Part model, mm, in its own coordinate system. Face numbers are marked on the shaded views. A direction names the side the tool comes from. Coordinates: 2 decimals unless noted, no trailing zeros. Loops run counter-clockwise (first coordinate to the right, second up) from the corner with the lowest first, then second, coordinate; pieces in that order, holes last.
Autodesk Inventor part; units mm, degrees
ref_plane "YZ Plane" through (0, 0, 0) normal (1, 0, 0) x (0, 1, 0)
ref_plane "XZ Plane" through (0, 0, 0) normal (0, 1, 0) x (-1, 0, 0)
ref_plane "XY Plane" through (0, 0, 0) normal (0, 0, 1) x (1, 0, 0)
sketch "Sketch1" plane through (0, 0, 0) normal (0, 0, 1) x (1, 0, 0)
  line L0 (-34.8609, 0) -> (34.8609, 0) construction
  line L1 (0, -34.8609) -> (0, 34.8609) construction
  line L2 (0, 0) -> (13.4339, 13.4339) construction
  line L3 (0, 0) -> (18.9985, 0) construction
  line L4 (0, 24.9006) -> (16.8, 24.9006)
  line L5 (16.8, 24.9006) -> (16.8, 21.2406)
  line L6 (16.8, 21.2406) -> (19.0203, 19.0203)
  line L7 (24.9006, 0) -> (24.9006, 16.8)
  line L8 (24.9006, 16.8) -> (21.2406, 16.8)
  line L9 (21.2406, 16.8) -> (19.0203, 19.0203)
  line L10 (0, 0) -> (-13.4339, 13.4339) construction
  line L11 (0, 0) -> (-18.9985, 0) construction
  line L12 (0, 24.9006) -> (-16.8, 24.9006)
  line L13 (-16.8, 24.9006) -> (-16.8, 21.2406)
  line L14 (-16.8, 21.2406) -> (-19.0203, 19.0203)
  line L15 (-24.9006, 0) -> (-24.9006, 16.8)
  line L16 (-24.9006, 16.8) -> (-21.2406, 16.8)
  line L17 (-21.2406, 16.8) -> (-19.0203, 19.0203)
  line L18 (0, 0) -> (13.4339, -13.4339) construction
  line L19 (0, -24.9006) -> (16.8, -24.9006)
  line L20 (16.8, -24.9006) -> (16.8, -21.2406)
  line L21 (16.8, -21.2406) -> (19.0203, -19.0203)
  line L22 (24.9006, 0) -> (24.9006, -16.8)
  line L23 (24.9006, -16.8) -> (21.2406, -16.8)
  line L24 (21.2406, -16.8) -> (19.0203, -19.0203)
  line L25 (0, 0) -> (-13.4339, -13.4339) construction
  line L26 (0, -24.9006) -> (-16.8, -24.9006)
  line L27 (-16.8, -24.9006) -> (-16.8, -21.2406)
  line L28 (-16.8, -21.2406) -> (-19.0203, -19.0203)
  line L29 (-24.9006, 0) -> (-24.9006, -16.8)
  line L30 (-24.9006, -16.8) -> (-21.2406, -16.8)
  line L31 (-21.2406, -16.8) -> (-19.0203, -19.0203)
  dimension "d0" = 45
  dimension "d1" = 3.14
  dimension "d2" = 3.66
  dimension "d3" = 16.8
extrude "Extrusion1" add sketch "Sketch1" along normal blind 5
hole "Hole1" at (0, 0, 0) direction (0, 0, 1) diameter 25.7 end through all
sketch "Sketch2" plane through (0, 0, 0) normal (0, 0, -1) x (-1, 0, 0)
  circle A0 centre (0, 0) radius 12.85
  line L0 (16.8, 24.9006) -> (-16.8, 24.9006)
  line L1 (-16.8, 24.9006) -> (-16.8, 21.2406)
  line L2 (-16.8, 21.2406) -> (-21.2406, 16.8)
  line L3 (-21.2406, 16.8) -> (-24.9006, 16.8)
  line L4 (-24.9006, 16.8) -> (-24.9006, -16.8)
  line L5 (-24.9006, -16.8) -> (-21.2406, -16.8)
  line L6 (-21.2406, -16.8) -> (-16.8, -21.2406)
  line L7 (-16.8, -21.2406) -> (-16.8, -24.9006)
  line L8 (-16.8, -24.9006) -> (16.8, -24.9006)
  line L9 (16.8, -24.9006) -> (16.8, -21.2406)
  line L10 (16.8, -21.2406) -> (21.2406, -16.8)
  line L11 (21.2406, -16.8) -> (24.9006, -16.8)
  line L12 (24.9006, -16.8) -> (24.9006, 16.8)
  line L13 (24.9006, 16.8) -> (21.2406, 16.8)
  line L14 (21.2406, 16.8) -> (16.8, 21.2406)
  line L15 (16.8, 21.2406) -> (16.8, 24.9006)
  circle A1 centre (0, 0) radius 11.85
  dimension "d17" = 1
extrude "Extrusion2" add sketch "Sketch2" against normal blind 1 contours A0
equation "\"Lens_diameter\" = 25"
properties part number "20_Lens_holder"
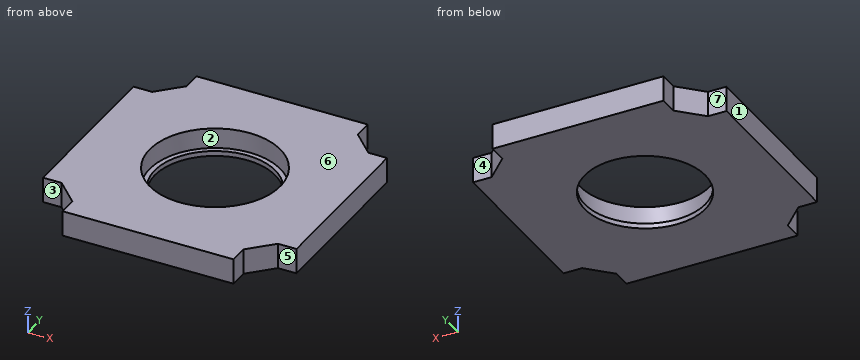
Q1. Saw through at D-D (x = -22). List the corners of the cut face in (y, z).
Q2. Saw through at A-A (z = 3.9). List the corners of the cut face in (x, y).
Q3. Mould opens along Y. For the marked faces 1, 2 and 3 say: released by +Y, released by -Y, zero draft, split by the parting line, or undercut.
Q4. Tool access for the marked faces 4, 5, 6 and 7: list every direction of +Z, -Z, +X, -X, +Y, -Y with a clear straight run to the whole face (end or side of a thin tool).
Q5. Probe line 1 (Y direction, x = 0, z = 0.2); line 2 (X direction, y = 0, z = 2). List the from-to ranges inside material, lowest first.
Q6. Drop flat-ended pins along their axis: P1, Ø1.8, axis at y = -23, z = 3, coming from the +X side; P2, Ø14, axis at x = 0, y = 0, coming from the +Z side; P3, Ø3, axis at y = 22.5, z = 3, coming from the +X side; P4, Ø1.1, axis at x = 23, z = 1.5, coming from the -Y side. Give the stop position or say it passes through.
Q7. Saw through at B-B (y = 0). List the corners of the cut face in (x, z).
Checked values:
1. outline: (-16.8, 0) - (16.8, 0) - (16.8, 5) - (-16.8, 5) - close
2. outline: (-24.9, -16.8) - (-21.24, -16.8) - (-16.8, -21.24) - (-16.8, -24.9) - (16.8, -24.9) - (16.8, -21.24) - (21.24, -16.8) - (24.9, -16.8) - (24.9, 16.8) - (21.24, 16.8) - (16.8, 21.24) - (16.8, 24.9) - (-16.8, 24.9) - (-16.8, 21.24) - (-21.24, 16.8) - (-24.9, 16.8) - close; hole circle Ø25.7 at (0, 0)
3. face 1: zero draft
3. face 2: undercut
3. face 3: released by -Y
4. face 4: +Z, -Z, +X, +Y
4. face 5: +Z, -Z, +X, -Y
4. face 6: +Z, +X, -X, +Y, -Y
4. face 7: +Z, -Z, -X, +Y
5. line 1: y = -24.9 to -11.85, 11.85 to 24.9
5. line 2: x = -24.9 to -12.85, 12.85 to 24.9
6. P1: stops at x = 16.8
6. P2: passes through
6. P3: stops at x = 17.04
6. P4: stops at y = -16.8
7. outline: (-24.9, 0) - (-11.85, 0) - (-11.85, 1) - (-12.85, 1) - (-12.85, 5) - (-24.9, 5) - close; (11.85, 0) - (24.9, 0) - (24.9, 5) - (12.85, 5) - (12.85, 1) - (11.85, 1) - close
